Design review of the part built by this model. Coordinates are the model's own, in mm. Give positions to 0.01 mm unless a question says otherwise; leave off trailing zeros. Loops run counter-clockwise (first coordinate to the right, second up) from the corner with the lowest first, then second, coordinate; pieces in that order, holes last. Notation, with made-up numbers: (70.25, -5) -> (88.25, -5) arc R21 ccw to (88.25, 11) -> close; hole circle Ø2 at (69, 56). An arc over 180 degrees is marked (long way). Answer in a Markdown table with one row per item. Add a question column.
(1) Consider section B-B on z = 0. Write out the cut boundary in (x, y), then the cut area to 3 significant figures.
(2) Draft analysis for pull direction Z (two halves, no side actions). For faces 1 (the cylindrical face through (1.532, 2.465, 4.864)), 2 (the cylindrical face through (98.563, 2.465, -4.575)), 3 (the cylindrical face through (20.32, 2.46, -4.51)), 4 (the cylindrical face through (68.489, 2.465, 20.015)), state which applies: +Z half, -Z half, draft (parallel to the pull), parting line (faces both ways), or undercut.
(3) For line 1 (X direction, y = 2.35, z = 0); line 2 (Z direction, x = 47, y = 1.35); line 3 (Z direction, x = 94, y = 4.6), list the stretches that pass through material, from the lowest coordinate up.
(4) For pin 1 (1.5 mm diameter, centred on x = 42, y = 1, fed in from +Z); pin 2 (3 mm diameter, centred on x = 21.5, y = 2, fed in from +Z); pin 3 (1.5 mm diameter, centred on y = 3, z = 18.5, fed in from -X), all flat-tipped, find the tip position at first contact; note any pin that passes through.
(5) Consider section D-D on z = 18. Write out the cut boundary in (x, y).
(6) Consider section A-A on x = 92. Write out the cut boundary in (y, z), then the cut area to 3 significant figures.
(7) Consider section C-C on y = 2.5. Count the separate pieces of the cut face and the enclosed holes in it, then the cut area to 3 significant figures.
from build123d import *

# Parameters (mm, degrees)
SKETCH_1_R      = 5.1
EXTRUDE_1_DEPTH = 5
FILLET_1_R      = 8


with BuildPart() as part:
    # 草图1 → 凸台-拉伸1 (new body)
    with BuildSketch(Plane(origin=(0, 0, 0), x_dir=(1, 0, 0), z_dir=(0, 1, 0))):
        with BuildLine():
            Line((-0.787870548, -7.961109219), (17.98227334, -9.818695034))
            Line((17.98227334, -9.818695034), (35.982367897, -22.422496932))
            ThreePointArc((35.982367897, -22.422496932), (67.859174016, -20.183513419), (96.717948718, -6.460724409))
            ThreePointArc((96.717948718, -6.460724409), (98.460724409, 4.717948718), (87.282051282, 6.460724409))
            ThreePointArc((87.282051282, 6.460724409), (64.699919143, -4.463945073), (39.716178923, -6.725320727))
            ThreePointArc((39.716178923, -6.725320727), (21.179057691, 4.200169373), (0, 8))
            ThreePointArc((0, 8), (-7.990271389, 0.394414913), (-0.787870548, -7.961109219))
        make_face()
        with Locations(Location((0, 0, 0), (0, 0, 270))):
            Circle(SKETCH_1_R, mode=Mode.SUBTRACT)
        with Locations(Location((92, 0, 0), (0, 0, 270))):
            Circle(SKETCH_1_R, mode=Mode.SUBTRACT)
    extrude(amount=EXTRUDE_1_DEPTH)

    # 圆角1
    fillet_1_edges = [part.edges().sort_by_distance(p)[0] for p in [
        (39.716178923, 2.5, 6.725320727),
        (35.982367897, 2.5, 22.422496932),
        (17.98227334, 2.5, 9.818695034),
    ]]
    fillet(fillet_1_edges, radius=FILLET_1_R)


solid = part.part
Values follow:
| question | item | result |
|---|---|---|
| 1 | outline | (-8, 0) -> (-5.1, 0) -> (-5.1, 5) -> (-8, 5) -> close; (5.1, 0) -> (30.18, 0) -> (30.18, 5) -> (5.1, 5) -> close; (76.53, 0) -> (86.9, 0) -> (86.9, 5) -> (76.53, 5) -> close; (97.1, 0) -> (100, 0) -> (100, 5) -> (97.1, 5) -> close |
| 1 | area | 206 mm2 |
| 2 | face 1 | undercut |
| 2 | face 2 | parting line |
| 2 | face 3 | -Z half |
| 2 | face 4 | +Z half |
| 3 | line 1 | -8 to -5.1, 5.1 to 30.18, 76.53 to 86.9, 97.1 to 100 |
| 3 | line 2 | 7 to 23 |
| 3 | line 3 | -7.75 to -4.69, 4.69 to 8.37 |
| 4 | pin 1 | z = 22.95 |
| 4 | pin 2 | z = 13.33 |
| 4 | pin 3 | x = 29.31 |
| 5 | outline | (29.67, 0) -> (74.92, 0) -> (74.92, 5) -> (29.67, 5) -> close |
| 6 | outline | (0, -8) -> (5, -8) -> (5, -5.1) -> (0, -5.1) -> close; (0, 5.1) -> (5, 5.1) -> (5, 9.67) -> (0, 9.67) -> close |
| 6 | area | 37.4 mm2 |
| 7 | separate pieces | 1 |
| 7 | enclosed holes | 2 |
| 7 | area | 1,590 mm2 |
